```python
from build123d import *

# Parameters (mm, degrees)
SKETCH1_W           = 60.96
SKETCH1_H           = 38.1
SKETCH1_W_2         = 48.26
SKETCH1_H_2         = 25.4
BOSS_EXTRUDE1_DEPTH = 9.525
SKETCH2_R           = 1.905
CUT_EXTRUDE1_DEPTH  = 64.883019849
FILLET1_R           = 6.35
FILLET2_R           = 1.5875


with BuildPart() as part:
    # Sketch1 → Boss-Extrude1 (new body)
    with BuildSketch(Plane(origin=(0, 0, 0), x_dir=(1, 0, 0), z_dir=(0, 1, 0))):
        with Locations((-24.13, -12.7)):
            Rectangle(SKETCH1_W, SKETCH1_H)
        with Locations((-24.13, -12.7)):
            Rectangle(SKETCH1_W_2, SKETCH1_H_2, mode=Mode.SUBTRACT)
    extrude(amount=BOSS_EXTRUDE1_DEPTH)

    # Sketch2 → Cut-Extrude1 (cut, through all)
    with BuildSketch(Plane.XY):
        with Locations((-36.83, 4.7625)):
            Circle(SKETCH2_R)
        with Locations((-11.43, 4.7625)):
            Circle(SKETCH2_R)
    extrude(amount=-CUT_EXTRUDE1_DEPTH, mode=Mode.SUBTRACT)

    # Fillet1
    fillet1_edges = [part.edges().sort_by_distance(p)[0] for p in [
        (-54.61, 4.7625, -6.35),
        (6.35, 4.7625, -6.35),
        (6.35, 4.7625, 31.75),
        (-54.61, 4.7625, 31.75),
    ]]
    fillet(fillet1_edges, radius=FILLET1_R)

    # Fillet2
    fillet2_edges = [part.edges().sort_by_distance(p)[0] for p in [
        (0, 0, 12.7),
        (0, 4.7625, 25.4),
        (-24.13, 0, 0),
        (0, 4.7625, 0),
        (-48.26, 0, 12.7),
        (-48.26, 4.7625, 0),
        (-24.13, 0, 25.4),
        (-48.26, 4.7625, 25.4),
        (0, 9.525, 12.7),
        (-24.13, 9.525, 0),
        (-48.26, 9.525, 12.7),
        (-24.13, 9.525, 25.4),
        (-24.13, 0, 31.75),
        (-24.13, 9.525, 31.75),
        (-54.61, 0, 12.7),
        (-24.13, 0, -6.35),
        (6.35, 0, 12.7),
        (4.490128061, 0, 29.890128061),
        (4.490128061, 0, -4.490128061),
        (-52.750128061, 0, -4.490128061),
        (-52.750128061, 0, 29.890128061),
        (-54.61, 9.525, 12.7),
        (6.35, 9.525, 12.7),
        (-24.13, 9.525, -6.35),
        (4.490128061, 9.525, 29.890128061),
        (4.490128061, 9.525, -4.490128061),
        (-52.750128061, 9.525, -4.490128061),
        (-52.750128061, 9.525, 29.890128061),
    ]]
    fillet(fillet2_edges, radius=FILLET2_R)


solid = part.part
```
Source: CAD feature listing. Evaluate the final solid. Frame: model axes, mm. A direction names the side the tool comes from. Round coordinates to 2 decimals unless told otherwise and drop trailing zeros.
1. Access query for faces 1 (the cylindrical face through (-13.333, 4.846, -3.131)), 2 (the flat face through (0, 5, 13)), 3 (the cylindrical face through (-23.814, 9.072, 25.877)). Directions: +Z, -Z, +X, -X, +Y, -Y. A direction counts if a zero-diameter tool reaches every point of the face in a straight line with its end or side. Return the directions, or none.
2. Mould query, pull axis Z, two halves, no side actions, for faces 4 (the flat face through (-24, 5, 25.4)), 5 (the cylindrical face through (-52.8, 4.81, 29.84)), 6 (the cylindrical face through (-52.8, 4.81, -4.44)). Classes: released by +Z, released by -Z, zero draft, split by the parting line, or undercut.
3. Contact query for flat-ended pins moving along their axis: pin 1 (5 mm diameter, centred on x = -12.5, z = 2, fed in from -Y); pin 2 (2.5 mm diameter, centred on x = -11.43, y = 4.76, fed in from -Z). Output: stop coordinate, or through.
4. Ray query, L1, parallel to X at y = 3.75, z = 9.5; L2, parallel to Y at x = -36.83, z = -1.75 (1 decimal); L3, parallel to Z at x = -20.5, y = 3.5. Return the intervals inside material, ascending.
5. Section query B-B on x = -11.43. Give the number of separate pieces and of enclosed holes in the cut face, and give its area (3 significant figures).
Answers below:
1. face 1: -Z
1. face 2: +Y, -Y
1. face 3: +Y
2. face 4: undercut
2. face 5: released by +Z
2. face 6: released by -Z
3. pin 1: stops at y = 0.43
3. pin 2: stops at z = 25.4
4. L1: x = -54.61 to -48.26, 0 to 6.35
4. L2: y = 0 to 2.9, 6.7 to 9.5
4. L3: z = -6.35 to 0, 25.4 to 31.75
5. separate pieces: 3
5. enclosed holes: 0
5. area: 92.4 mm2
